Part model, mm, in its own coordinate system. Round coordinates to 2 decimals unless told otherwise and drop trailing zeros. Loops run counter-clockwise (first coordinate to the right, second up) from the corner with the lowest first, then second, coordinate; pieces in that order, holes last.
(1) Cut at B-B on x = -12.5. List the corners of the cut face in (y, z), then the cut area to 3 significant figures.
(2) Probe probe 1 along X at (y, z) = (2.6, -21); probe 2 along Z at (x, y) = (-12, 3.2); probe 3 along Z at (x, y) = (3, 3.6). List the from-to ranges inside material, lowest first.
(3) Mould opens along Z. For faces 1 (the face through (-16.89, 2.54, 14.85)), 2 (the face through (12.57, 2.46, -20.75)), 3 (the face through (8, 5, -13)) say: +Z half, -Z half, draft (parallel to the pull), parting line (faces both ways), or undercut.
(4) Cut at C-C on y = 1.5. List the corners of the cut face in (x, z), then the cut area to 3 significant figures.
(5) Cut at D-D on z = 7.75. List the corners of the cut face in (x, y).
(6) Cut at A-A on x = 0. List the corners of the cut face in (y, z), then the cut area to 3 significant figures.
from build123d import *

# Parameters (mm, degrees)
SKETCH_1_W          = 35.5
SKETCH_1_H          = 46
SKETCH_1_R          = 8.2
EXTRUDE_1_DEPTH     = 5
FILLET_2_R          = 3
SKETCH_3_R          = 1.5
CUT_EXTRUDE_1_DEPTH = 10


with BuildPart() as part:
    # 草图1 → 凸台-拉伸1 (new body)
    with BuildSketch(Plane(origin=(0, 0, 0), x_dir=(1, 0, 0), z_dir=(0, 1, 0))):
        with Locations((0, 7.25)):
            Rectangle(SKETCH_1_W, SKETCH_1_H)
        with Locations(Location((0, 7.25, 0), (0, 0, 270))):
            Circle(SKETCH_1_R, mode=Mode.SUBTRACT)
    extrude(amount=EXTRUDE_1_DEPTH)

    # 圆角2
    fillet_2_edges = [part.edges().sort_by_distance(p)[0] for p in [
        (-17.75, 2.5, -30.25),
        (17.75, 2.5, -30.25),
        (17.75, 2.5, 15.75),
        (-17.75, 2.5, 15.75),
    ]]
    fillet(fillet_2_edges, radius=FILLET_2_R)

    # 草图3 → 切除-拉伸1 (cut)
    with BuildSketch(Plane.XZ):
        with Locations(Location((-12.5, 7.75, 0), (0, 0, 270))):
            Circle(SKETCH_3_R)
        with Locations(Location((12.5, 7.75, 0), (0, 0, 270))):
            Circle(SKETCH_3_R)
        with Locations(Location((12.5, -22.25, 0), (0, 0, 270))):
            Circle(SKETCH_3_R)
        with Locations(Location((-12.5, -22.25, 0), (0, 0, 270))):
            Circle(SKETCH_3_R)
    extrude(amount=-CUT_EXTRUDE_1_DEPTH, mode=Mode.SUBTRACT)


solid = part.part
Final values:
1. outline: (0, -30.25) - (5, -30.25) - (5, -23.75) - (0, -23.75) - close; (0, -20.75) - (5, -20.75) - (5, 6.25) - (0, 6.25) - close; (0, 9.25) - (5, 9.25) - (5, 15.75) - (0, 15.75) - close
1. area: 200 mm2
2. probe 1: x = -17.75 to -13.33, -11.67 to 11.67, 13.33 to 17.75
2. probe 2: z = -30.25 to -23.66, -20.84 to 6.34, 9.16 to 15.75
2. probe 3: z = -30.25 to -14.88, 0.38 to 15.75
3. face 1: +Z half
3. face 2: undercut
3. face 3: draft
4. outline: (-17.75, -27.25) arc R3 ccw to (-14.75, -30.25) - (14.75, -30.25) arc R3 ccw to (17.75, -27.25) - (17.75, 12.75) arc R3 ccw to (14.75, 15.75) - (-14.75, 15.75) arc R3 ccw to (-17.75, 12.75) - close; hole circle Ø3 at (-12.5, -22.25); hole circle Ø3 at (-12.5, 7.75); hole circle Ø16.4 at (0, -7.25); hole circle Ø3 at (12.5, -22.25); hole circle Ø3 at (12.5, 7.75)
4. area: 1,390 mm2
5. outline: (-17.75, 0) - (-14, 0) - (-14, 5) - (-17.75, 5) - close; (-11, 0) - (11, 0) - (11, 5) - (-11, 5) - close; (14, 0) - (17.75, 0) - (17.75, 5) - (14, 5) - close
6. outline: (0, -30.25) - (5, -30.25) - (5, -15.45) - (0, -15.45) - close; (0, 0.95) - (5, 0.95) - (5, 15.75) - (0, 15.75) - close
6. area: 148 mm2
